```python
from build123d import *

# Parameters (mm, degrees)
SM_BASE_FLANGE_1_DEPTH       = 52
CUT_EXTRUDE_1_REACH          = 100.25
SKETCH_6_R                   = 3
HOLE_WIZARD_M3_2_D           = 2.5
HOLE_WIZARD_M3_2_DEPTH       = 7.5
HOLE_WIZARD_M3_2_CBORE_D     = 3
HOLE_WIZARD_M3_2_CBORE_DEPTH = 6
HOLE_WIZARD_M3_2_TIP         = 0.751075774
SKETCH_9_W                   = 22
SKETCH_9_H                   = 42
CUT_EXTRUDE_2_DEPTH          = 10
SKETCH_10_W                  = 40
SKETCH_10_H                  = 14.2634
EXTRUDE_4_DEPTH              = 2
FILLET_1_R                   = 4


# Sheet-metal steps are written as plain solids
with BuildPart() as part:
    # Sketch 1 → 基材-凸緣1 (new body)
    with BuildSketch(Plane.XY):
        with BuildLine():
            Line((0, 80), (0, 0.7366))
            ThreePointArc((0, 0.7366), (0.215745145, 0.215745145), (0.7366, 0))
            Line((0.7366, 0), (15, 0))
            Line((15, 0), (15, -2))
            Line((15, -2), (0.7366, -2))
            ThreePointArc((0.7366, -2), (-1.198468417, -1.198468417), (-2, 0.7366))
            Line((-2, 0.7366), (-2, 80))
            Line((-2, 80), (0, 80))
        make_face()
    extrude(amount=SM_BASE_FLANGE_1_DEPTH)

    # 草圖6 → 除料-伸長1 (cut, up to next)
    with BuildSketch(Plane.XZ.offset(2), mode=Mode.PRIVATE) as cut_extrude_1_sk1:
        with Locations(Location((9, 26, 0), (0, 0, 270))):
            Circle(SKETCH_6_R)
    cut_extrude_1_tool1 = extrude(cut_extrude_1_sk1.sketch, amount=-CUT_EXTRUDE_1_REACH, mode=Mode.PRIVATE) & part.part
    add(cut_extrude_1_tool1.solids().sort_by_distance((9, -2, 26))[0], mode=Mode.SUBTRACT)

    # M3 螺紋孔2
    with Locations(Plane.ZY.offset(2)):
        with Locations((21, 61), (21, 13), (31, 13), (31, 61), (3.5, 76.5), (48.5, 76.5)):
            CounterBoreHole(HOLE_WIZARD_M3_2_D / 2, HOLE_WIZARD_M3_2_CBORE_D / 2, HOLE_WIZARD_M3_2_CBORE_DEPTH, depth=HOLE_WIZARD_M3_2_DEPTH)
            with Locations((0, 0, -(HOLE_WIZARD_M3_2_DEPTH + HOLE_WIZARD_M3_2_TIP / 2))):  # 118° drill point
                Cone(0, HOLE_WIZARD_M3_2_D / 2, HOLE_WIZARD_M3_2_TIP, mode=Mode.SUBTRACT)

    # 草圖9 → 除料-伸長2 (cut)
    with BuildSketch(Plane(origin=(0, 0, 0), x_dir=(0, 0, -1), z_dir=(1, 0, 0))):
        with Locations((-26, 37)):
            Rectangle(SKETCH_9_W, SKETCH_9_H)
    extrude(amount=-CUT_EXTRUDE_2_DEPTH, mode=Mode.SUBTRACT)

    # 草圖10 → 填料-伸長4 (add)
    with BuildSketch(Plane.ZX.offset(-2)):
        with Locations((72, 7.8683)):
            Rectangle(SKETCH_10_W, SKETCH_10_H)
    extrude(amount=EXTRUDE_4_DEPTH)

    # 圓角1
    fillet_1_edges = [part.edges().sort_by_distance(p)[0] for p in [
        (0.7366, -1, 92),
        (15, -1, 92),
    ]]
    fillet(fillet_1_edges, radius=FILLET_1_R)


solid = part.part
```
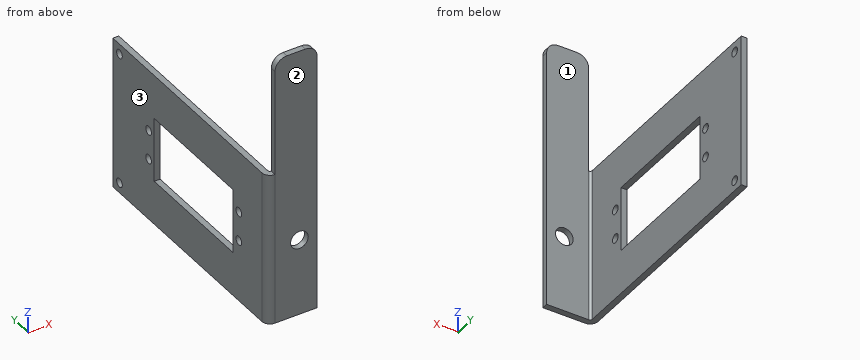
Geometry check sheet. Reference: the model listing, model coordinates, mm. Face numbers are marked on the shaded views. Give positions to 0.01 mm unless a question says otherwise; leave off trailing zeros. Order: outer loops, then holes, each group sorted by start corner. A loop starts at its lowest first (then second) coordinate and runs counter-clockwise, first axis right, second up. Notation, with made-up numbers: (-17.75, 16) - (-11.75, 16) arc R20 cw to (-11.75, 39) - close; hole circle Ø8 at (67, 69.5). An arc over 180 degrees is marked (long way). Write item = value, one per line. Start each with the question number.
1) Draft check along Y on the marked faces 1, 2 and 3. Enter one of: released by +Y, released by -Y, zero draft, split by the parting line, or undercut.
2) Section check A-A (z = 3.5). Enter the section's corners in (x, y), then the cut area to 3 significant figures.
3) Section check C-C (z = 21). Enter the section's corners in (x, y).
4) Scan lines: L1, parallel to Z at x = -0.8, y = 76.5; L2, parallel to X at y = 64, z = 28.5. Record each from-to range of solid material in increasing order.
5) Section check B-B (x = 9). Enter the section's corners in (y, z).
6) Gauge pin test, flat ends, axial feed: pin 1 Ø1 at (x, z) = (13, 19) entering from +Y; pin 2 Ø1 at (x, z) = (-1.5, 30.5) entering from -Y; pin 3 Ø6 at (y, z) = (17, 16.5) entering from +X. Record the tip position at first contact, or that the pin passes through.
7) Section check D-D (y = 27.5). Enter the section's corners in (x, z), then the cut area to 3 significant figures.
Geometry check:
q1.face_1 = released by +Y
q1.face_2 = released by -Y
q1.face_3 = zero draft
q2.outline = (-2, 0.74) arc R2.74 ccw to (0.74, -2) - (15, -2) - (15, 0) - (0.74, 0) arc R0.74 cw to (0, 0.74) - (0, 75) - (-2, 75) - close; (-2, 78) - (0, 78) - (0, 80) - (-2, 80) - close
q2.area = 187 mm2
q3.outline = (-2, 0.74) arc R2.74 ccw to (0.74, -2) - (15, -2) - (15, 0) - (0.74, 0) arc R0.74 cw to (0, 0.74) - (0, 11.5) - (-2, 11.5) - close; (-2, 14.5) - (0, 14.5) - (0, 16) - (-2, 16) - close; (-2, 58) - (0, 58) - (0, 59.5) - (-2, 59.5) - close; (-2, 62.5) - (0, 62.5) - (0, 80) - (-2, 80) - close
q4.L1 = 0 to 2, 5 to 47, 50 to 52
q4.L2 = -2 to 0
q5.outline = (-2, 0) - (0, 0) - (0, 23) - (-2, 23) - close; (-2, 29) - (0, 29) - (0, 92) - (-2, 92) - close
q6.pin_1 = 0
q6.pin_2 = -1.38
q6.pin_3 = 0
q7.outline = (-2, 0) - (0, 0) - (0, 15) - (-2, 15) - close; (-2, 37) - (0, 37) - (0, 52) - (-2, 52) - close
q7.area = 60.0 mm2
